```python
from build123d import *

# Parameters (mm, degrees)
SKETCH1_R           = 60
BOSS_EXTRUDE1_DEPTH = 3
CUT_EXTRUDE1_REACH  = 86.906
SKETCH2_R           = 3.5
SKETCH2_R_2         = 1.8
SKETCH3_R           = 54
SKETCH3_R_2         = 36
BOSS_EXTRUDE2_DEPTH = 3


with BuildPart() as part:
    # Sketch1 → Boss-Extrude1 (new body)
    with BuildSketch(Plane(origin=(0, 0, 0), x_dir=(1, 0, 0), z_dir=(0, 1, 0))):
        with Locations(Location((0, 0, 0), (0, 0, 270))):
            Circle(SKETCH1_R)
    extrude(amount=BOSS_EXTRUDE1_DEPTH)

    # Sketch2 → Cut-Extrude1 (cut, up to next)
    with BuildSketch(Plane.XZ, mode=Mode.PRIVATE) as cut_extrude1_sk1:
        with Locations(Location((0, 0, 0), (0, 0, 270))):
            Circle(SKETCH2_R)
    cut_extrude1_tool1 = extrude(cut_extrude1_sk1.sketch, amount=-CUT_EXTRUDE1_REACH, mode=Mode.PRIVATE) & part.part
    # Sketch2 → Cut-Extrude1 (cut, up to next)
    with BuildSketch(Plane.XZ, mode=Mode.PRIVATE) as cut_extrude1_sk2:
        with Locations(Location((1.56993281, 6.821679483, 0), (0, 0, 270))):
            Circle(SKETCH2_R_2)
    cut_extrude1_tool2 = extrude(cut_extrude1_sk2.sketch, amount=-CUT_EXTRUDE1_REACH, mode=Mode.PRIVATE) & part.part
    # Sketch2 → Cut-Extrude1 (cut, up to next)
    with BuildSketch(Plane.XZ, mode=Mode.PRIVATE) as cut_extrude1_sk3:
        with Locations(Location((6.821679483, -1.56993281, 0), (0, 0, 270))):
            Circle(SKETCH2_R_2)
    cut_extrude1_tool3 = extrude(cut_extrude1_sk3.sketch, amount=-CUT_EXTRUDE1_REACH, mode=Mode.PRIVATE) & part.part
    # Sketch2 → Cut-Extrude1 (cut, up to next)
    with BuildSketch(Plane.XZ, mode=Mode.PRIVATE) as cut_extrude1_sk4:
        with Locations(Location((-1.56993281, -6.821679483, 0), (0, 0, 270))):
            Circle(SKETCH2_R_2)
    cut_extrude1_tool4 = extrude(cut_extrude1_sk4.sketch, amount=-CUT_EXTRUDE1_REACH, mode=Mode.PRIVATE) & part.part
    # Sketch2 → Cut-Extrude1 (cut, up to next)
    with BuildSketch(Plane.XZ, mode=Mode.PRIVATE) as cut_extrude1_sk5:
        with Locations(Location((-6.821679483, 1.56993281, 0), (0, 0, 270))):
            Circle(SKETCH2_R_2)
    cut_extrude1_tool5 = extrude(cut_extrude1_sk5.sketch, amount=-CUT_EXTRUDE1_REACH, mode=Mode.PRIVATE) & part.part
    add(cut_extrude1_tool1.solids().sort_by_distance((0, 0, 0))[0], mode=Mode.SUBTRACT)
    add(cut_extrude1_tool2.solids().sort_by_distance((1.569933, 0, 6.821679))[0], mode=Mode.SUBTRACT)
    add(cut_extrude1_tool3.solids().sort_by_distance((6.821679, 0, -1.569933))[0], mode=Mode.SUBTRACT)
    add(cut_extrude1_tool4.solids().sort_by_distance((-1.569933, 0, -6.821679))[0], mode=Mode.SUBTRACT)
    add(cut_extrude1_tool5.solids().sort_by_distance((-6.821679, 0, 1.569933))[0], mode=Mode.SUBTRACT)

    # Sketch3 → Boss-Extrude2 (add)
    with BuildSketch(Plane.XZ):
        with Locations(Location((0, 0, 0), (0, 0, 90))):
            Circle(SKETCH3_R)
        with Locations(Location((0, 0, 0), (0, 0, 270))):
            Circle(SKETCH3_R_2, mode=Mode.SUBTRACT)
    extrude(amount=BOSS_EXTRUDE2_DEPTH)


solid = part.part
```
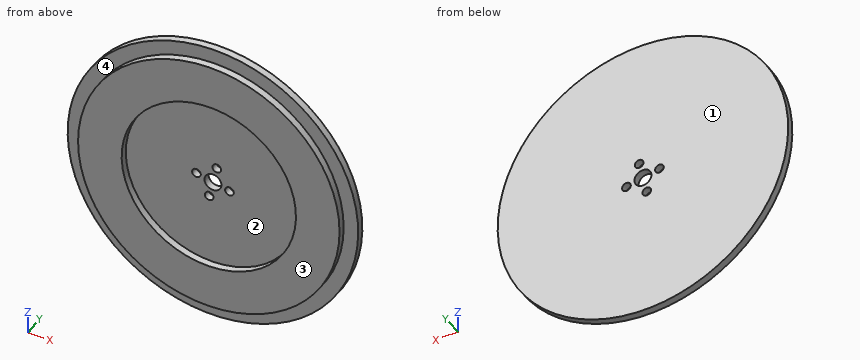
The listing builds one solid part. Answer for the finished solid, in the listing's coordinates (mm). Face numbers are marked on the shaded views. A direction names the side the tool comes from. Give positions to 0.01 mm unless a question says otherwise; leave off trailing zeros. Order: outer loops, then holes, each group sorted by start corner. A loop starts at its lowest first (then second) coordinate and runs counter-clockwise, first axis right, second up.
1) Find section C-C on z = -27.5. Write down the section's boundary in (x, y).
Reported:
outline: (-53.33, 0) - (-46.47, 0) - (-46.47, -3) - (-23.23, -3) - (-23.23, 0) - (23.23, 0) - (23.23, -3) - (46.47, -3) - (46.47, 0) - (53.33, 0) - (53.33, 3) - (-53.33, 3) - close
2) Given P1, Ø1.5, axis at x = -30.5, y = -1, coming from the +Z side; P2, Ø2, axis at y = 1, z = 13, coming from the +X side; P3, Ø1, axis at x = -18, z = -13, coming from the -Y side, each flat-ended and moving along its own axis, determine where each tip first touches the part or whether it passes through.
Reported:
P1: stops at z = 45.07
P2: stops at x = 58.79
P3: stops at y = 0
3) Find section B-B on y = -1.75. Write down the section's boundary in (x, z).
Reported:
outline: circle Ø108 at (0, 0); hole circle Ø72 at (0, 0)
4) For the marked faces 3 and 4, determine the directions among +Z, -Z, +X, -X, +Y, -Y from which every point of the face is accessible in a straight line to the end or side of a thin tool.
Reported:
face 3: +Z, -Z, +X, -X, -Y
face 4: -Y
5) Determine the mould class of the marked faces 1 and 2 for opening direction Z: pulls with the +Z half, pulls with the -Z half, needs draft (parallel to the pull), parting line crosses it, or undercut.
Reported:
face 1: needs draft
face 2: undercut
6) Consider line 1 along Z through (x, y) = (0.5, -2.2); line 2 along Y through (x, z) = (11.5, 20). Determine where each line is inside the solid, lowest interval first.
Reported:
line 1: z = -54 to -36, 36 to 54
line 2: y = 0 to 3
7) Find section A-A on x = -22. Write down the section's boundary in (y, z), then the cut area to 3 significant figures.
Reported:
outline: (-3, -49.32) - (0, -49.32) - (0, -55.82) - (3, -55.82) - (3, 55.82) - (0, 55.82) - (0, 49.32) - (-3, 49.32) - (-3, 28.5) - (0, 28.5) - (0, -28.5) - (-3, -28.5) - close
area: 460 mm2
